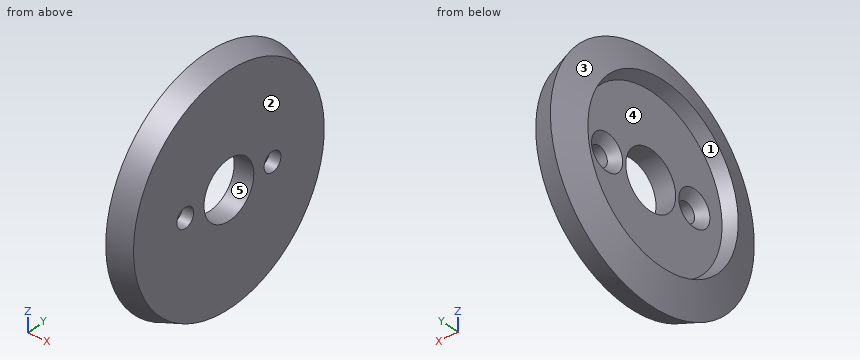
from build123d import *

# Parameters (mm, degrees)
CSK_FOR_M3_FLAT_COUNTERSUNK_HEAD_SCREW1_D           = 2.7
CSK_FOR_M3_FLAT_COUNTERSUNK_HEAD_SCREW1_CSINK_D     = 5
CSK_FOR_M3_FLAT_COUNTERSUNK_HEAD_SCREW1_CSINK_ANGLE = 90


with BuildPart() as part:
    # Sketch1 → Revolve1 (revolve)
    with BuildSketch(Plane(origin=(0, 0, 0), x_dir=(-1, 0, 0), z_dir=(0, 0, -1)), mode=Mode.PRIVATE) as revolve1_sk:
        Polygon((-9.95, 4), (-7.190575715, 4), (-7.190575715, 11.457942816), (-5.45, 12.070691824), (-6.96, 16.36), (-9.95, 15.307406012), align=None)
    revolve(revolve1_sk.sketch.rotate(Axis((15.476540881, 0, 0), (-1, 0, 0)), 270), axis=Axis((15.476540881, 0, 0), (-1, 0, 0)))

    # CSK for M3 Flat Countersunk Head Screw1 (through all)
    with Locations(Plane.ZY.offset(-7.190575715)):
        with Locations((0, 7), (0, -7)):
            CounterSinkHole(CSK_FOR_M3_FLAT_COUNTERSUNK_HEAD_SCREW1_D / 2, CSK_FOR_M3_FLAT_COUNTERSUNK_HEAD_SCREW1_CSINK_D / 2, counter_sink_angle=CSK_FOR_M3_FLAT_COUNTERSUNK_HEAD_SCREW1_CSINK_ANGLE)


solid = part.part
CAD build for the part. Positions are in the model's coordinates, mm. Face numbers are marked on the shaded views. A direction names the side the tool comes from. Round coordinates to 2 decimals unless told otherwise and drop trailing zeros. Write each loop counter-clockwise with the first axis right and the second up, starting at its lowest first coordinate (ties: lowest second). Pieces come first, ordered by that corner, then holes.
(1) Slice it at C-C, the plane x = 6.45. Write the cut outline in (y, z).
(2) 3-axis set-ups, long thin cutter, end or side, ignore diameter. For the marked faces 4 and 5: which of +Z, -Z, +X, -X, +Y, -Y reach the whole face in a straight line?
(3) Mould opens along Z. For the marked faces 1, 2 and 3 say: pulls with the +Z half, pulls with the -Z half, needs draft (parallel to the pull), parting line crosses it, or undercut.
(4) Slice it at D-D, the plane x = 9.25. Write the cut outline in (y, z), and give its area (3 significant figures).
(5) Slice it at B-B, the plane z = 0. Write the cut outline in (x, y).
(6) Slice it at A-A, the plane y = 0. Write the cut outline in (x, z), and give its area (3 significant figures).
(7) Probe line 1 along Y through (x, z) = (9.45, 0.5); line 2 along Y through (x, z) = (9.65, 0); line 3 along X through (y, z) = (6, -3). List the from-to ranges inside material, lowest first.
(8) Drop flat-ended pins along their axis: P1, Ø1.5, axis at x = 7, y = -5.5, coming from the -Z side; P2, Ø11.5, axis at y = 4.5, z = -1.5, coming from the -X side. Give the stop position or say it passes through.
From the geometry:
1. outline: circle Ø29.82 at (0, 0); hole circle Ø23.44 at (0, 0)
2. face 4: -X
2. face 5: +X, -X
3. face 1: undercut
3. face 2: needs draft
3. face 3: parting line crosses it
4. outline: circle Ø31.11 at (0, 0); hole circle Ø2.7 at (-7, 0); hole circle Ø8 at (0, 0); hole circle Ø2.7 at (7, 0)
4. area: 698 mm2
5. outline: (5.45, -12.07) - (6.96, -16.36) - (9.95, -15.31) - (9.95, -8.35) - (8.34, -8.35) - (7.19, -9.5) - (7.19, -11.46) - close; (5.45, 12.07) - (7.19, 11.46) - (7.19, 9.5) - (8.34, 8.35) - (9.95, 8.35) - (9.95, 15.31) - (6.96, 16.36) - close; (7.19, -4.5) - (8.34, -5.65) - (9.95, -5.65) - (9.95, -4) - (7.19, -4) - close; (7.19, 4) - (9.95, 4) - (9.95, 5.65) - (8.34, 5.65) - (7.19, 4.5) - close
6. outline: (5.45, -12.07) - (6.96, -16.36) - (9.95, -15.31) - (9.95, -4) - (7.19, -4) - (7.19, -11.46) - close; (5.45, 12.07) - (7.19, 11.46) - (7.19, 4) - (9.95, 4) - (9.95, 15.31) - (6.96, 16.36) - close
6. area: 74.6 mm2
7. line 1: y = -15.48 to -8.25, -5.75 to -3.97, 3.97 to 5.75, 8.25 to 15.48
7. line 2: y = -15.41 to -8.35, -5.65 to -4, 4 to 5.65, 8.35 to 15.41
7. line 3: x = 7.19 to 9.95
8. P1: stops at z = -15.65
8. P2: stops at x = 7.19
